Can you work these out from the model? Positions are in its coordinate system, mm. Face numbers are marked on the shaded views. A direction names the side the tool comes from. Give positions to 0.01 mm unless a question says otherwise; leave off trailing zeros. Order: outer loops, then holes, each group sorted by start corner. A loop starts at its lowest first (then second) coordinate and runs counter-clockwise, first axis right, second up. Notation, with made-up numbers: (46, -39.5) - (74, -39.5) arc R10 ccw to (74, -24.5) - close; hole circle Ø9 at (54.25, -39.75). An arc over 180 degrees is marked (long way). Return JSON: item names as keys, results as strings.
```python
from build123d import *

# Parameters (mm, degrees)
BOSS_EXTRUDE1_DEPTH = 1
FILLET2_R           = 2.5
SKETCH4_R           = 2
CUT_EXTRUDE1_DEPTH  = 34.047536431


with BuildPart() as part:
    # Sketch1 → Boss-Extrude1 (new body)
    with BuildSketch(Plane(origin=(0, 0, 0), x_dir=(1, 0, 0), z_dir=(0, 1, 0))):
        with BuildLine():
            Line((-2.306769174, 23.799171975), (-12.34435681, 9.4640112))
            ThreePointArc((-12.34435681, 9.4640112), (-15.328348079, 0), (-12.34435681, -9.4640112))
            Line((-12.34435681, -9.4640112), (-2.306769174, -23.799171975))
            ThreePointArc((-2.306769174, -23.799171975), (0, -25), (2.306769174, -23.799171975))
            Line((2.306769174, -23.799171975), (12.34435681, -9.4640112))
            ThreePointArc((12.34435681, -9.4640112), (15.328348079, 0), (12.34435681, 9.4640112))
            Line((12.34435681, 9.4640112), (2.306769174, 23.799171975))
            ThreePointArc((2.306769174, 23.799171975), (0, 25), (-2.306769174, 23.799171975))
        make_face()
    extrude(amount=BOSS_EXTRUDE1_DEPTH)

    # Sketch3 → Revolve1 (revolve)
    with BuildSketch(Plane.XY, mode=Mode.PRIVATE) as revolve1_sk:
        with BuildLine():
            Line((0, 1), (12, 1))
            Line((12, 1), (12, 13))
            ThreePointArc((12, 13), (10.06934138, 15.353606271), (7.156329697, 16.2375))
            Line((7.156329697, 16.2375), (4.656329697, 16.2375))
            ThreePointArc((4.656329697, 16.2375), (3.704315473, 12.244265441), (0, 10.475))
            Line((0, 10.475), (0, 1))
        make_face()
    revolve(revolve1_sk.sketch.rotate(Axis((0, 10.475, 0), (0, -1, 0)), 90), axis=Axis((0, 10.475, 0), (0, -1, 0)))

    # Fillet2
    fillet2_edges = [part.edges().sort_by_distance(p)[0] for p in [
        (0, 13, -12),
    ]]
    fillet(fillet2_edges, radius=FILLET2_R)

    # Sketch4 → Cut-Extrude1 (cut, through all)
    with BuildSketch(Plane(origin=(0, 1, 0), x_dir=(1, 0, 0), z_dir=(0, 1, 0))):
        with Locations(Location((0, -22.18395481, 0), (0, 0, 270))):
            Circle(SKETCH4_R)
        with Locations(Location((0, 22.18395481, 0), (0, 0, 270))):
            Circle(SKETCH4_R)
    extrude(amount=-CUT_EXTRUDE1_DEPTH, mode=Mode.SUBTRACT)


solid = part.part
```
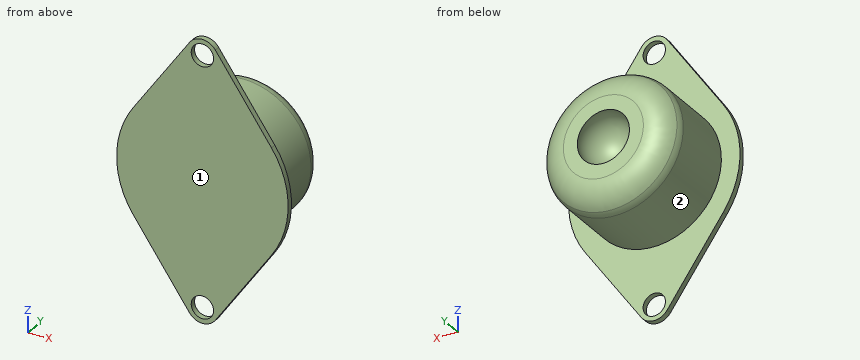
1. Suppose I cut it at D-D (z = -18). List the corners of the cut face in (x, y) for me.
Checks:
{"outline": "(-6.37, 0) - (6.37, 0) - (6.37, 1) - (-6.37, 1) - close"}
2. On a 3-axis mill with a long thin cutter (end or side, diameter ignored), from which of +Z, -Z, +X, -X, +Y, -Y can I reach the whole of each face in a straight line? I mean the marked faces 1 and 2. Say none if no direction works.
Checks:
{"face 1": "+Z, -Z, +X, -X, -Y", "face 2": "+Y"}
3. Suppose I cut it at A-A (y = 3.75). List the corners of the cut face in (x, z) for me, plus the area to 3 significant figures.
Checks:
{"outline": "circle Ø24 at (0, 0)", "area": "452 mm^2"}
4. For pin 1 Ø1 at (y, z) = (12, -2) entering from +X; pin 2 Ø4 at (x, y) = (2, 3.5) entering from -Z; pin 3 Ø3 at (x, z) = (0, -22.18) entering from +Y; pin 4 Ø6 at (x, y) = (-4.5, 7.5) entering from +Z, each with a flat end and sliding along its axis, tell me the tip position at first contact or that it passes through.
Checks:
{"pin 1": "x = 11.91", "pin 2": "z = -12", "pin 3": "through", "pin 4": "z = 11.91"}
5. If I drill on L1, parallel to Y at x = 0, z = -18.5; L2, parallel to X at y = 3.75, z = -0.5; L3, parallel to X at y = 10.25, z = 8, over which ranges is the centre line in solid material (lowest first)? Write a range as [from, to].
Checks:
{"L1": "[0, 1]", "L2": "[-11.99, 11.99]", "L3": "[-8.94, 8.94]"}
6. Suppose I cut it at C-C (y = 14.75). List the corners of the cut face in (x, z) for me, plus the area to 3 significant figures.
Checks:
{"outline": "circle Ø21.63 at (0, 0); hole circle Ø9.47 at (0, 0)", "area": "297 mm^2"}
7. Suppose I cut it at B-B (x = 0). State how many separate pieces and enclosed holes the cut face has, plus the area to 3 significant figures.
Checks:
{"separate pieces": "3", "enclosed holes": "0", "area": "354 mm^2"}
